```python
from build123d import *

# Parameters (mm, degrees)
SKETCH1_W           = 9.8
SKETCH1_H           = 59.5
BOSS_EXTRUDE1_DEPTH = 2
SKETCH2_W           = 9.8
SKETCH2_H           = 64
BOSS_EXTRUDE2_DEPTH = 1
FILLET1_R           = 3
BOSS_EXTRUDE3_DEPTH = 2
SKETCH4_R           = 2
BOSS_EXTRUDE4_DEPTH = 3
FILLET2_R           = 3
FILLET3_R           = 3
SKETCH5_R           = 2
BOSS_EXTRUDE5_DEPTH = 3
FILLET4_R           = 10
FILLET6_R           = 3
FILLET7_R           = 3
BOSS_EXTRUDE6_DEPTH = 3
CHAMFER1_SIZE2      = 3
CHAMFER1_SIZE       = 17.013845459
FILLET10_R          = 3
CUT_EXTRUDE1_DEPTH  = 117.582838676
BOSS_EXTRUDE7_DEPTH = 2
SKETCH9_R           = 1.7
CUT_EXTRUDE2_DEPTH  = 117.582838676
CHAMFER2_SIZE       = 1


# Some blends are built 0.0001 mm under size
with BuildPart() as part:
    # Sketch1 → Boss-Extrude1 (new body)
    with BuildSketch(Plane(origin=(0, 0, 0), x_dir=(0, 0, -1), z_dir=(1, 0, 0))):
        with Locations((41.694735288, 0)):
            Rectangle(SKETCH1_W, SKETCH1_H)
    extrude(amount=BOSS_EXTRUDE1_DEPTH)

    # Sketch2 → Boss-Extrude2 (add)
    with BuildSketch(Plane(origin=(0, 0, 0), x_dir=(0, 0, -1), z_dir=(1, 0, 0))):
        with Locations((41.694735288, 0)):
            Rectangle(SKETCH2_W, SKETCH2_H)
    extrude(amount=BOSS_EXTRUDE2_DEPTH)

    # Fillet1
    fillet1_edges = [part.edges().sort_by_distance(p)[0] for p in [
        (0.5, -32, -46.594735288),
        (0.5, 32, -46.594735288),
    ]]
    fillet(fillet1_edges, radius=FILLET1_R)

    # Sketch3 → Boss-Extrude3 (add)
    with BuildSketch(Plane(origin=(0, 0, 0), x_dir=(0, 0, -1), z_dir=(1, 0, 0))):
        Polygon((36.794735288, 29.75), (-63.205264712, 43), (-103.205264712, 43), (-103.205264712, -43), (-63.205264712, -43), (36.794735288, -29.75), align=None)
    extrude(amount=BOSS_EXTRUDE3_DEPTH)

    # Sketch4 → Boss-Extrude4 (add)
    with BuildSketch(Plane.XY.offset(103.205264712)):
        with BuildLine():
            Line((2, -43), (-9, -43))
            ThreePointArc((-9, -43), (-11.121320344, -42.121320344), (-12, -40))
            Line((-12, -40), (-12, -34))
            ThreePointArc((-12, -34), (-11.121320344, -31.878679656), (-9, -31))
            Line((-9, -31), (-7, -31))
            ThreePointArc((-7, -31), (-2.050252532, -28.949747468), (0, -24))
            Line((0, -24), (0, -23))
            Line((0, -23), (2, -23))
            Line((2, -23), (2, -31))
            Line((2, -31), (2, -43))
        make_face()
        with Locations((-6, -37)):
            Circle(SKETCH4_R, mode=Mode.SUBTRACT)
    extrude(amount=BOSS_EXTRUDE4_DEPTH)

    # Fillet2
    fillet2_edges = [part.edges().sort_by_distance(p)[0] for p in [
        (1, -23, 103.205264712),
    ]]
    fillet(fillet2_edges, radius=FILLET2_R - 0.0001)  # a hair under: the kernel refuses the full size

    # Fillet3
    # the kernel refuses this fillet: 3 mm, written as the material it takes off along each edge
    with BuildSketch(Plane(origin=(-5.490486718, -23, 106.205264712), x_dir=(0, 0.2587982993664488, -0.9659313848535175), z_dir=(1, 0, 0))) as fillet3_piece_1:
        with BuildLine():
            CenterArc((2.329422704, -2.897768274), FILLET3_R, 105.000679234, 60.000551337)
            Line((-0.56837145, -2.121373376), (-0.858150866, -2.043733886))
            Line((-0.858150866, -2.043733886), (-0.289779415, 0.07763949))
            Line((-0.289779415, 0.07763949), (0.07763949, 0.289779415))
            ThreePointArc((0.07763949, 0.289779415), (0.077736083, 0.289753536), (1.475282068, 0.289776827))
            Line((1.475282068, 0.289776827), (1.552931216, 0))
        make_face()
    extrude(amount=12.980973437, mode=Mode.SUBTRACT)

    # Sketch5 → Boss-Extrude5 (add)
    with BuildSketch(Plane.XY.offset(103.205264712)):
        with BuildLine():
            Line((-8, 33), (-9, 33))
            ThreePointArc((-9, 33), (-11.121320344, 32.121320344), (-12, 30))
            Line((-12, 30), (-12, 24))
            ThreePointArc((-12, 24), (-11.121320344, 21.878679656), (-9, 21))
            Line((-9, 21), (-8, 21))
            ThreePointArc((-8, 21), (-2.343145751, 18.656854249), (0, 13))
            Line((0, 13), (0, 12.9))
            Line((0, 12.9), (2, 12.9))
            Line((2, 12.9), (2, 21))
            Line((2, 21), (2, 33))
            Line((2, 33), (2, 43))
            Line((2, 43), (0, 43))
            Line((0, 43), (0, 41))
            ThreePointArc((0, 41), (-2.343145751, 35.343145751), (-8, 33))
        make_face()
        with Locations((-6, 27)):
            Circle(SKETCH5_R, mode=Mode.SUBTRACT)
    extrude(amount=BOSS_EXTRUDE5_DEPTH)

    # Fillet4
    # the kernel refuses this fillet: 10 mm, written as the material it takes off along each edge
    with BuildSketch(Plane(origin=(27, 43, 106.205264712), x_dir=(0, 0, -1), z_dir=(-1, 0, 0))) as fillet4_piece_1:
        with BuildLine():
            CenterArc((FILLET4_R, FILLET4_R), FILLET4_R, 180, 90)
            Line((0, FILLET4_R), (0, 0))
            Line((0, 0), (FILLET4_R, 0))
        make_face()
    extrude(amount=52, mode=Mode.SUBTRACT)

    # Fillet6
    fillet6_edges = [part.edges().sort_by_distance(p)[0] for p in [
        (1, 12.9, 103.205264712),
    ]]
    fillet(fillet6_edges, radius=FILLET6_R - 0.0001)  # a hair under: the kernel refuses the full size

    # Fillet7
    # the kernel refuses this fillet: 3 mm, written as the material it takes off along each edge
    with BuildSketch(Plane(origin=(-5.490486718, 12.9, 106.205264712), x_dir=(0, -0.2587982993664468, -0.9659313848535179), z_dir=(1, 0, 0))) as fillet7_piece_1:
        with BuildLine():
            CenterArc((2.329422704, 2.897768274), FILLET7_R, 194.99876943, 60.000551337)
            Line((-0.56837145, 2.121373376), (-0.858150866, 2.043733886))
            Line((-0.858150866, 2.043733886), (-0.289779415, -0.07763949))
            Line((-0.289779415, -0.07763949), (0.07763949, -0.289779415))
            ThreePointArc((0.07763949, -0.289779415), (0.077736083, -0.289753536), (1.475282068, -0.289776827))
            Line((1.475282068, -0.289776827), (1.552931216, 0))
        make_face()
    extrude(amount=12.980973437, mode=Mode.SUBTRACT)

    # Sketch6 → Boss-Extrude6 (add)
    with BuildSketch(Plane.XZ.offset(43)):
        Polygon((2, 106.205264712), (-9, 106.205264712), (-9, 103.205264712), (0, 76.205264712), (2, 76.205264712), align=None)
    extrude(amount=BOSS_EXTRUDE6_DEPTH)

    # Chamfer1
    chamfer1_edges = [part.edges().sort_by_distance(p)[0] for p in [
        (1, -46, 76.205264712),
    ]]
    chamfer1_side = [part.faces().sort_by_distance(p)[0] for p in [
        (1, -46, 76.265264712),
    ]]
    chamfer(chamfer1_edges, length=CHAMFER1_SIZE - 0.0001, length2=CHAMFER1_SIZE2 - 0.0001, reference=chamfer1_side[0])  # a hair under: the kernel refuses the full size

    # Fillet10
    fillet10_edges = [part.edges().sort_by_distance(p)[0] for p in [
        (2, -46, 99.712137442),
        (-3.5, -46, 106.205264712),
    ]]
    fillet(fillet10_edges, radius=FILLET10_R)

    # Sketch7 → Cut-Extrude1 (cut, through all)
    with BuildSketch(Plane(origin=(2, 0, 0), x_dir=(0, 0, -1), z_dir=(1, 0, 0))):
        Polygon((35.650666719, 21.831669631), (35.650666719, -21.798973174), (-62.72810878, -34.834160927), (-95.091144317, -34.834160927), (-95.091144317, 34.834160927), (-62.481343063, 34.834160927), align=None)
    extrude(amount=-CUT_EXTRUDE1_DEPTH, mode=Mode.SUBTRACT)

    # Sketch8 → Boss-Extrude7 (add)
    with BuildSketch(Plane(origin=(2, 0, 0), x_dir=(0, 0, -1), z_dir=(1, 0, 0))):
        Polygon((-78.78624369, 34.834160927), (-37.27250726, 0), (-78.78624369, -34.834160927), (-66.340453075, -34.834160927), (-31.049611953, -5.221629157), (-4.891583353, -27.170821308), (-1.562241162, -29.964471113), (8.678277132, -28.114027922), (5.856936901, -25.746642374), (-24.826716646, 0), (5.856936901, 25.746642374), (7.77511163, 27.665346604), (-2.902361224, 28.796551739), (-4.891583353, 27.170821308), (-31.049611953, 5.221629157), (-66.340453075, 34.834160927), align=None)
    extrude(amount=-BOSS_EXTRUDE7_DEPTH)

    # Sketch9 → Cut-Extrude2 (cut, through all)
    with BuildSketch(Plane(origin=(2, 0, 0), x_dir=(0, 0, -1), z_dir=(1, 0, 0))):
        with Locations((42.594735288, 24)):
            Circle(SKETCH9_R)
        with Locations((42.594735288, -24)):
            Circle(SKETCH9_R)
    extrude(amount=-CUT_EXTRUDE2_DEPTH, mode=Mode.SUBTRACT)

    # Chamfer2
    chamfer2_edges = [part.edges().sort_by_distance(p)[0] for p in [
        (2, 24, -40.894735288),
        (2, -24, -40.894735288),
    ]]
    chamfer(chamfer2_edges, length=CHAMFER2_SIZE)


solid = part.part
```
The listing builds one solid part. Answer for the finished solid, in the listing's coordinates (mm). A direction names the side the tool comes from. Give positions to 0.01 mm unless a question says otherwise; leave off trailing zeros. Write each loop counter-clockwise with the first axis right and the second up, starting at its lowest first coordinate (ties: lowest second). Pieces come first, ordered by that corner, then holes. Notation, with made-up numbers: M 59,5 L 64,5 A19 cw 64,31 Z; hole C 66,46 d6. An arc over 180 degrees is marked long. Write each question's results on one line, items separated by ' | '.
Q1. Flat-ended cylindrical pins translate along their axes: P1, Ø2, axis at x = 1.5, z = 85.5, coming from the -Y side; P2, Ø4, axis at x = -1, z = 34.5, coming from the -Y side; P3, Ø1, axis at x = -1.5, z = 3.5, coming from the +Y side; P4, Ø12, axis at y = 24, z = 71.5, coming from the -X side. Find the tip coordinate at first contact, or state that the pin passes through.
Output values:
P1: y = -44.81 | P2: y = -39.43 | P3: through | P4: x = 0
Q2. Consider L1, parallel to Y at x = 0.75, z = 51.5; L2, parallel to Z at x = 1.75, y = -9; L3, parallel to Y at x = -6, z = 105.3. Determine where each line is inside the solid, lowest interval first. Write a range as from..to.
Output values:
L1: -41.45..-33.35, -22.38..-11.94, 11.94..22.38, 33.38..41.45 | L2: -46.59..-35.65, 14.1..26.55, 35.55..48, 95.09..103.21 | L3: -45.15..-39, -35..-30.93, 20.75..25, 29..33.25
Q3. For a pull along Y with two mould halves and no side action, classify faces 1 (the cylindrical face through (-2.1, -29, 104.7)), 2 (the flat face through (-12, 27, 105)), 3 (the cylindrical face through (-11.1, 32.14, 104.68)) as released by +Y, released by -Y, zero draft, split by the parting line, or undercut.
Output values:
face 1: undercut | face 2: zero draft | face 3: released by +Y
Q4. Section A-A, the plane z = 14.5 is taken. Write down the section's boundary in (x, y).
Output values:
outline: M 0,-36.55 L 2,-36.55 L 2,-28.44 L 0,-28.44 Z; M 0,-19.11 L 2,-19.11 L 2,-8.67 L 0,-8.67 Z; M 0,8.67 L 2,8.67 L 2,19.11 L 0,19.11 Z; M 0,28.48 L 2,28.48 L 2,36.55 L 0,36.55 Z
Q5. Section C-C, the plane z = -28 is taken. Write down the section's boundary in (x, y).
Output values:
outline: M 0,-30.92 L 2,-30.92 L 2,-22.81 L 0,-22.81 Z; M 0,22.85 L 2,22.85 L 2,30.92 L 0,30.92 Z
Q6. Section B-B, the plane y = -37 is taken. Write down the section's boundary in (x, z).
Output values:
outline: M -12,103.21 L -8,103.21 L -8,106.21 L -12,106.21 Z; M -4,103.21 L 0,103.21 L 0,17.92 L 2,17.92 L 2,106.21 L -4,106.21 Z
Q7. A tool of negligible diameter and unlimited length cuts with its end or side. For faces 4 (the cylindrical face through (-11.14, -31.9, 104.68)), 5 (the cylindrical face through (0.57, 30.694, -46.071)), 6 (the flat face through (0.986, 36.282, 12.505)), 7 (the flat face through (1.014, -23.745, -20.962)), from which of +Z, -Z, +X, -X, +Y, -Y can it reach the whole face along a straight path? Write none if from no direction.
Output values:
face 4: +Z, -Z, -X | face 5: -Z, +X, -X, +Y | face 6: +X, -X, +Y | face 7: +X, -X
